The model under review builds one solid part; all positions refer to its coordinate system, in mm. A direction names the side the tool comes from. Coordinates: 2 decimals unless noted, no trailing zeros. Write each loop counter-clockwise with the first axis right and the second up, starting at its lowest first coordinate (ties: lowest second). Pieces come first, ordered by that corner, then holes.
1) For line 1 (X direction, y = 7, z = 109); line 2 (Y direction, x = 26.5, z = 109); line 3 (X direction, y = 15, z = 91), list the stretches that pass through material, from the lowest coordinate up.
2) Add section D-D, the plane x = 159.5. State the section outline as (y, z) points, then the cut area to 3 significant figures.
3) For P1, Ø1.8, axis at x = 2, y = 15.5, coming from the -Z side; P2, Ø4, axis at x = 31, z = 38, coming from the +Y side, all flat-tipped, find the tip position at first contact; note any pin that passes through.
4) Add section C-C, the plane z = 146. State the section outline as (x, y) points, then the cut area to 3 significant figures.
5) Machinability: for faces 5 (the flat face through (80, 15, 156)), 6 (the flat face through (87, 15, 80)), 7 (the flat face through (132.33, 0.99, 30)), which of the approach directions +Z, -Z, +X, -X, +Y, -Y give a long, thin tool a straight path to every point of the face, cutting with its end or side? Answer none if there is none.
6) Mouldability with a two-part tool opening along X and no side actions: class faces 1 (the flat face through (94, 0, 118)), 2 (the flat face through (2, 6, 114)), 3 (the flat face through (57.67, 30.01, 55)), 4 (the flat face through (190, 15, 114)) as released by +X, released by -X, zero draft, split by the parting line, or undercut.
7) Add section A-A, the plane z = 65. State the section outline as (x, y) points, then the cut area to 3 significant figures.
8) Add section B-B, the plane x = 20. State the section outline as (y, z) points, then the cut area to 3 significant figures.
from build123d import *

# Parameters (mm, degrees)
F0_W     = 190
F0_H     = 31
F0_R     = 1.5
F1_DEPTH = 232
F2_W     = 2
F2_H     = 150
F2_H_2   = 2
F2_W_2   = 17
F3_DEPTH = 29.5
F4_W     = 160
F4_H     = 47
F5_DEPTH = 5
F6_W     = 160
F6_H     = 22
F7_DEPTH = 5
F8_R     = 10


with BuildPart() as f1:
    # F0 (on Top) → F1 (new body)
    with BuildSketch(Plane.XY):
        with Locations((95, 15.5)):
            Rectangle(F0_W, F0_H)
        with Locations((2, 15.5)):
            Circle(F0_R, mode=Mode.SUBTRACT)
        Polygon((188, 2), (2, 2), (2, 10.3786796564), (5, 13.3786796564), (5, 17.6213203436), (2, 20.6213203436), (2, 29), (188, 29), (188, 20.6213203436), (185, 17.6213203436), (185, 13.3786796564), (188, 10.3786796564), align=None, mode=Mode.SUBTRACT)
        with Locations((188, 15.5)):
            Circle(F0_R, mode=Mode.SUBTRACT)
    extrude(amount=F1_DEPTH)

    # F2 (on face) → F3 (join)
    with BuildSketch(Plane.XZ):
        with Locations((79, 157)):
            Rectangle(F2_W, F2_H)
        with Locations((79, 81)):
            Rectangle(F2_W, F2_H_2)
        with Locations((88.5, 81)):
            Rectangle(F2_W_2, F2_H_2)
    extrude(amount=-F3_DEPTH)

    # F4 (on face) → F5 (cut)
    with BuildSketch(Plane(origin=(0, 31, 0), x_dir=(-1, 0, 0), z_dir=(0, 1, 0))):
        Polygon((-95, 62), (-175, 47), (-15, 47), align=None)
        with Locations((-95, 23.5)):
            Rectangle(F4_W, F4_H)
    extrude(amount=-F5_DEPTH, mode=Mode.SUBTRACT)

    # F6 (on face) → F7 (cut)
    with BuildSketch(Plane.XZ):
        Polygon((95, 37), (15, 22), (175, 22), align=None)
        with Locations((95, 11)):
            Rectangle(F6_W, F6_H)
    extrude(amount=-F7_DEPTH, mode=Mode.SUBTRACT)

    # F8
    f8_edges = [f1.edges().sort_by_distance(p)[0] for p in [
        (15, 30, 47),
        (15, 1, 22),
        (175, 30, 47),
        (175, 1, 22),
        (95, 30, 62),
        (95, 1, 37),
    ]]
    fillet(f8_edges, radius=F8_R)


solid = f1.part
Geometry results:
1. line 1: x = 0 to 2, 78 to 80, 188 to 190
1. line 2: y = 0 to 2, 29 to 31
1. line 3: x = 0 to 0.59, 3.41 to 5, 78 to 80, 185 to 186.59, 189.41 to 190
2. outline: (0, 24.91) - (2, 24.91) - (2, 232) - (0, 232) - close; (29, 49.91) - (31, 49.91) - (31, 232) - (29, 232) - close
2. area: 778 mm2
3. P1: passes through
3. P2: stops at y = 2
4. outline: (0, 0) - (190, 0) - (190, 31) - (0, 31) - close; hole circle Ø3 at (2, 15.5); hole (2, 2) - (78, 2) - (78, 29) - (2, 29) - (2, 20.62) - (5, 17.62) - (5, 13.38) - (2, 10.38) - close; hole (80, 2) - (188, 2) - (188, 10.38) - (185, 13.38) - (185, 17.62) - (188, 20.62) - (188, 29) - (80, 29) - close; hole circle Ø3 at (188, 15.5)
4. area: 951 mm2
5. face 5: +Z
5. face 6: -Z
5. face 7: -Z, +Y, -Y
6. face 1: zero draft
6. face 2: undercut
6. face 3: undercut
6. face 4: released by +X
7. outline: (0, 0) - (190, 0) - (190, 31) - (0, 31) - close; hole circle Ø3 at (2, 15.5); hole (2, 2) - (188, 2) - (188, 10.38) - (185, 13.38) - (185, 17.62) - (188, 20.62) - (188, 29) - (2, 29) - (2, 20.62) - (5, 17.62) - (5, 13.38) - (2, 10.38) - close; hole circle Ø3 at (188, 15.5)
7. area: 897 mm2
8. outline: (0, 22.36) - (2, 22.36) - (2, 232) - (0, 232) - close; (29, 47.36) - (31, 47.36) - (31, 232) - (29, 232) - close
8. area: 789 mm2
